Part print with two shaded views. Sizes in mm from the minimum x, y, z corner. A direction names the side the tool comes from. Coordinates: 2 decimals unless noted, no trailing zeros. Loops run counter-clockwise (first coordinate to the right, second up) from the corner with the lowest first, then second, coordinate; pieces in that order, holes last. Notation, with made-up numbers: (54.5, -1.75) -> (93.5, -1.75) arc R15 cw to (93.5, 17.25) -> close; hole circle Ø11 at (-1, 31). An arc over 180 degrees is marked (long way). Answer as a JSON object with one key per item and string values. Group by question number.
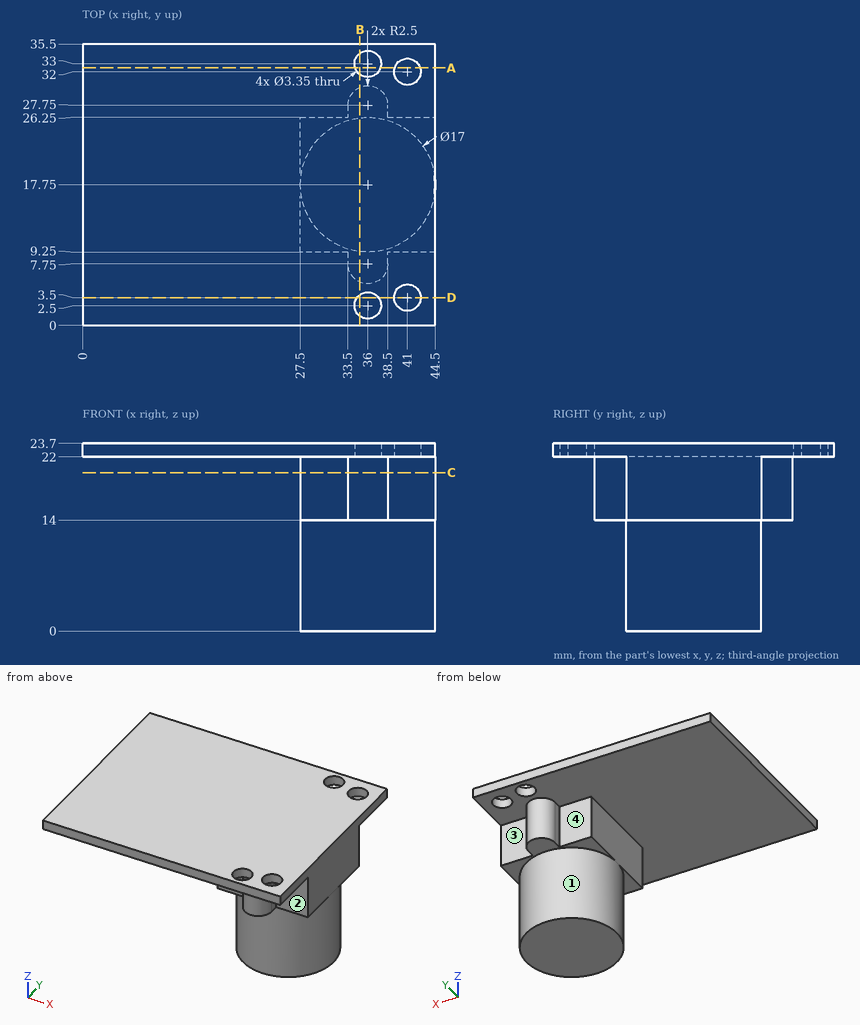
Item 1: Band-saw the part on A-A, the plane y = 32.5. List the corners of the cut face in (x, z).
Item 2: Band-saw the part on D-D, the plane y = 3.5. List the corners of the cut face in (x, z) (3 decimals), and give its area (3 significant figures).
Item 3: Band-saw the part on C-C, the plane z = 20. List the corners of the cut face in (x, y), and give its area (3 significant figures).
Item 4: 3-axis set-ups, long thin cutter, end or side, ignore diameter. For the marked faces 1, 2, 3 and 4: which of +Z, -Z, +X, -X, +Y, -Y reach the whole face in a straight line?
Item 5: Drill centre lines: L1, parallel to Y at x = 41, z = 22.6 (3 decimals); L2, parallel to Y at x = 36, z = 22.6 (3 decimals); L3, parallel to X at y = 2.5, z = 23.25 (3 decimals). Where is each one in solid material? Low to high.
Item 6: Flat gauge pins, fed straight in: P1, Ø1, axis at x = 31.5, y = 6.5, coming from the -Z side; P2, Ø3, axis at x = 30.5, z = 18, coming from the -Y side; P3, Ø6, axis at y = 31, z = 11.5, coming from the +X side; P4, Ø3, axis at x = 41, y = 3.5, coming from the -Z side. Where does each tip first touch, or does it go through?
Item 7: Band-saw the part on B-B, the plane x = 35. List the corners of the cut face in (y, z).
Reply:
{
 "1": {"outline": "(0, 22) -> (34.4, 22) -> (34.4, 23.7) -> (0, 23.7) -> close; (37.6, 22) -> (39.4, 22) -> (39.4, 23.7) -> (37.6, 23.7) -> close; (42.6, 22) -> (44.5, 22) -> (44.5, 23.7) -> (42.6, 23.7) -> close"},
 "2": {"outline": "(0, 22) -> (34.656, 22) -> (34.656, 23.7) -> (0, 23.7) -> close; (37.344, 22) -> (39.325, 22) -> (39.325, 23.7) -> (37.344, 23.7) -> close; (42.675, 22) -> (44.5, 22) -> (44.5, 23.7) -> (42.675, 23.7) -> close", "area": "65.4 mm²"},
 "3": {"outline": "(27.5, 9.25) -> (33.5, 9.25) -> (33.5, 7.75) arc R2.5 ccw to (38.5, 7.75) -> (38.5, 9.25) -> (44.5, 9.25) -> (44.5, 26.25) -> (38.5, 26.25) -> (38.5, 27.75) arc R2.5 ccw to (33.5, 27.75) -> (33.5, 26.25) -> (27.5, 26.25) -> close", "area": "324 mm²"},
 "4": {"face 1": "-Z", "face 2": "-Z, +X, -Y", "face 3": "-Z, +X, +Y", "face 4": "-Z, -X, +Y"},
 "5": {"L1": "0 to 1.825, 5.175 to 30.325, 33.675 to 35.5", "L2": "0 to 0.825, 4.175 to 31.325, 34.675 to 35.5", "L3": "0 to 34.325, 37.675 to 39.656, 42.344 to 44.5"},
 "6": {"P1": "z = 22", "P2": "y = 9.25", "P3": "x = 37.93", "P4": "through"},
 "7": {"outline": "(0, 22) -> (1.16, 22) -> (1.16, 23.7) -> (0, 23.7) -> close; (3.84, 22) -> (5.46, 22) -> (5.46, 14) -> (9.31, 14) -> (9.31, 0) -> (26.19, 0) -> (26.19, 14) -> (30.04, 14) -> (30.04, 22) -> (31.66, 22) -> (31.66, 23.7) -> (3.84, 23.7) -> close; (34.34, 22) -> (35.5, 22) -> (35.5, 23.7) -> (34.34, 23.7) -> close"}
}
